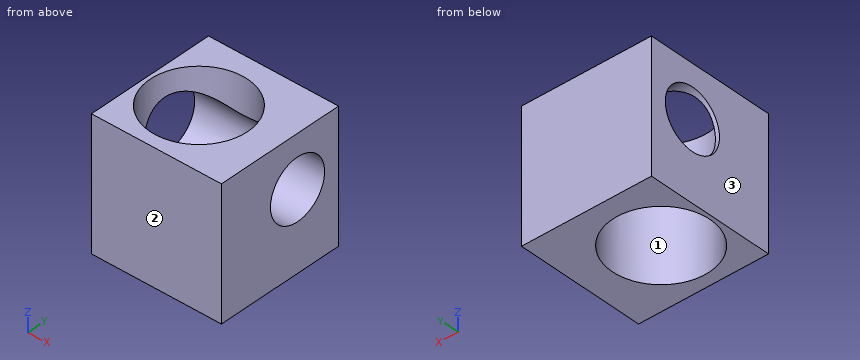
from build123d import *

# Parameters (mm, degrees)
F0_W     = 100
F0_H     = 100
F1_DEPTH = 100
F2_R     = 37.4790948787
F3_DEPTH = 100.001
F4_R     = 23.1250184434
F5_DEPTH = 100.001


with BuildPart() as f1:
    # F0 (on Top) → F1 (new body)
    with BuildSketch(Plane.XY):
        with Locations((-1.539904009, 9.2580467463)):
            Rectangle(F0_W, F0_H)
    extrude(amount=F1_DEPTH)

    # F2 (on face) → F3 (cut, through all)
    with BuildSketch(Plane.XY.offset(100)):
        with Locations((-11.2805515528, 6.312854588)):
            Circle(F2_R)
    extrude(amount=-F3_DEPTH, mode=Mode.SUBTRACT)

    # F4 (on face) → F5 (cut, through all)
    with BuildSketch(Plane(origin=(-51.539904009, 0, 0), x_dir=(0, -1, 0), z_dir=(-1, 0, 0))):
        with Locations((-24.2580467463, 60)):
            Circle(F4_R)
    extrude(amount=-F5_DEPTH, mode=Mode.SUBTRACT)


solid = f1.part
Geometry check sheet. Reference: the model listing, model coordinates, mm. Face numbers are marked on the shaded views. Give positions to 0.01 mm unless a question says otherwise; leave off trailing zeros. Order: outer loops, then holes, each group sorted by start corner. A loop starts at its lowest first (then second) coordinate and runs counter-clockwise, first axis right, second up.
1. Sectioned sample at C-C (z = 60). Record the boundary of the cut face in (x, y), then the cut area to 3 significant figures.
Completed:
outline: (-51.54, -40.74) - (48.46, -40.74) - (48.46, 1.13) - (25.84, 1.13) arc R37.48 cw to (-48.4, 1.13) - (-51.54, 1.13) - close; (-51.54, 47.38) - (48.46, 47.38) - (48.46, 59.26) - (-51.54, 59.26) - close
area: 3,560 mm2
2. Scan lines: line 1 (X direction, y = 6.5, z = 93); line 2 (Y direction, x = 16, z = 5.5); line 3 (Y direction, x = -15, z = 27). Record each from-to range of solid material in increasing order.
Completed:
line 1: x = -51.54 to -48.76, 26.2 to 48.46
line 2: y = -40.74 to -19.39, 32.01 to 59.26
line 3: y = -40.74 to -30.98, 43.61 to 59.26
3. Draft check along X on the marked faces 1, 2 and 3. Enter one of: pulls with the +X half, pulls with the -X half, needs draft (parallel to the pull), parting line crosses it, or undercut.
Completed:
face 1: undercut
face 2: needs draft
face 3: pulls with the -X half
4. Depth check by flat-ended pin: pin 1 (5 mm diameter, centred on x = 29.5, y = -4, fed in from -Z). Enter the tip coordinate at first touch or a pass-through.
Completed:
pin 1: stops at z = 0
5. Sectioned sample at D-D (z = 89). Record the boundary of the cut face in (x, y), then the cut area to 3 significant figures.
Completed:
outline: (-51.54, -40.74) - (48.46, -40.74) - (48.46, 59.26) - (-51.54, 59.26) - close; hole circle Ø74.96 at (-11.28, 6.31)
area: 5,590 mm2
6. Sectioned sample at A-A (y = 35). Record the boundary of the cut face in (x, z), then the cut area to 3 significant figures.
Completed:
outline: (-51.54, 0) - (-35.4, 0) - (-35.4, 39.52) - (-51.54, 39.52) - close; (-51.54, 80.48) - (-35.4, 80.48) - (-35.4, 100) - (-51.54, 100) - close; (12.84, 0) - (48.46, 0) - (48.46, 39.52) - (12.84, 39.52) - close; (12.84, 80.48) - (48.46, 80.48) - (48.46, 100) - (12.84, 100) - close
area: 3,060 mm2
7. Sectioned sample at B-B (x = -38). Record the boundary of the cut face in (y, z).
Completed:
outline: (-40.74, 0) - (-19.97, 0) - (-19.97, 100) - (-40.74, 100) - close; (32.6, 0) - (59.26, 0) - (59.26, 100) - (32.6, 100) - (32.6, 81.57) arc R23.13 cw to (32.6, 38.43) - close
